```python
from build123d import *

# Parameters (mm, degrees)
SKICA1_W                = 60
SKICA1_H                = 36
SKICA1_W_2              = 26
SKICA1_H_2              = 25
P_IDAT_VYSUNUT_M1_DEPTH = 1.2
SKICA2_W                = 10
SKICA2_H                = 10
P_IDAT_VYSUNUT_M2_DEPTH = 1.4
P_IDAT_VYSUNUT_M3_DEPTH = 6
M4_D_RA_S_V_L_1_D       = 4.5
ZAOBLIT1_R              = 2


with BuildPart() as part:
    # Skica1 → Přidat vysunutím1 (new body)
    with BuildSketch(Plane.XY):
        Rectangle(SKICA1_W, SKICA1_H)
        Rectangle(SKICA1_W_2, SKICA1_H_2, mode=Mode.SUBTRACT)
    extrude(amount=P_IDAT_VYSUNUT_M1_DEPTH)

    # Skica2 → Přidat vysunutím2 (add)
    with BuildSketch(Plane.XY.offset(1.2)):
        with Locations((22.5, 0)):
            Rectangle(SKICA2_W, SKICA2_H)
        with Locations((-22.5, 0)):
            Rectangle(SKICA2_W, SKICA2_H)
    extrude(amount=P_IDAT_VYSUNUT_M2_DEPTH)

    # Skica3 → Přidat vysunutím3 (add)
    with BuildSketch(Plane.XY.offset(1.2)):
        Polygon((-28.8, -16.8), (-28.8, 16.8), (-5, 16.8), (-5, 18), (-30, 18), (-30, -18), (-5, -18), (-5, -16.8), align=None)
        Polygon((28.8, -16.8), (5, -16.8), (5, -18), (30, -18), (30, 18), (5, 18), (5, 16.8), (28.8, 16.8), align=None)
    extrude(amount=P_IDAT_VYSUNUT_M3_DEPTH)

    # M4 díra s vůlí1 (through all)
    with Locations(Plane.XY.offset(2.6)):
        with Locations((-22.5, 0), (22.5, 0)):
            Hole(M4_D_RA_S_V_L_1_D / 2)

    # Zaoblit1
    zaoblit1_edges = [part.edges().sort_by_distance(p)[0] for p in [
        (30, -18, 3.6),
        (-30, -18, 3.6),
        (-30, 18, 3.6),
        (30, 18, 3.6),
    ]]
    fillet(zaoblit1_edges, radius=ZAOBLIT1_R)


solid = part.part
```
Source: CAD feature listing. Evaluate the final solid. Frame: model axes, mm. A direction names the side the tool comes from. Give positions to 0.01 mm unless a question says otherwise; leave off trailing zeros. Loops run counter-clockwise (first coordinate to the right, second up) from the corner with the lowest first, then second, coordinate; pieces in that order, holes last. Notation, with made-up numbers: (85, -12) - (142, -12) arc R33 cw to (142, 24) - close; hole circle Ø7 at (-8, 42.5). An arc over 180 degrees is marked (long way). Use CSV: the item, a comma, the result in double quotes.
1) Pin query (flat end, axial travel): P1, Ø1.3, axis at y = -17.5, z = 5.5, coming from the -X side; P2, Ø6, axis at x = -23, y = -7, coming from the +Z side; P3, Ø18, axis at x = -8.5, y = -6.5, coming from the +Z side; P4, Ø3.5, axis at x = 22.5, y = 0, coming from the +Z side. Return the tip coordinate at first contact, or that it passes through.
Worked out:
P1,"stops at x = -29.81"
P2,"stops at z = 2.6"
P3,"stops at z = 1.2"
P4,"passes through"
2) Mould query, pull axis X, two halves, no side actions, for faces 1 (the flat face through (17, -16.8, 4)), 2 (the flat face through (20, 0, 2.6)), 3 (the flat face through (-30, 0, 4)), 4 (the flat face through (0, -18, 1)). Classes: +X half, -X half, draft (parallel to the pull), parting line (faces both ways), or undercut.
Worked out:
face 1,"undercut"
face 2,"undercut"
face 3,"-X half"
face 4,"draft"
3) Line query: line 1 (Y direction, x = -26.5, z = 1.75); line 2 (X direction, y = -3.5, z = 2.25); line 3 (Y direction, x = -18.5, z = 6.5). Output: solid intervals per line, ascending.
Worked out:
line 1,"y = -18 to -16.8, -5 to 5, 16.8 to 18"
line 2,"x = -30 to -28.8, -27.5 to -17.5, 17.5 to 27.5, 28.8 to 30"
line 3,"y = -18 to -16.8, 16.8 to 18"
4) Cut plane B-B (y = 7.5). Output: boundary loops of the cut face in (x, z), and give its area (3 significant figures).
Worked out:
outline,"(-30, 0) - (-13, 0) - (-13, 1.2) - (-28.8, 1.2) - (-28.8, 7.2) - (-30, 7.2) - close; (13, 0) - (30, 0) - (30, 7.2) - (28.8, 7.2) - (28.8, 1.2) - (13, 1.2) - close"
area,"55.2 mm^2"
5) Cut plane C-C (x = -7.5). Output: boundary loops of the cut face in (y, z).
Worked out:
outline,"(-18, 0) - (-12.5, 0) - (-12.5, 1.2) - (-16.8, 1.2) - (-16.8, 7.2) - (-18, 7.2) - close; (12.5, 0) - (18, 0) - (18, 7.2) - (16.8, 7.2) - (16.8, 1.2) - (12.5, 1.2) - close"
6) Cut plane D-D (y = 0). Output: boundary loops of the cut face in (x, z).
Worked out:
outline,"(-30, 0) - (-24.75, 0) - (-24.75, 2.6) - (-27.5, 2.6) - (-27.5, 1.2) - (-28.8, 1.2) - (-28.8, 7.2) - (-30, 7.2) - close; (-20.25, 0) - (-13, 0) - (-13, 1.2) - (-17.5, 1.2) - (-17.5, 2.6) - (-20.25, 2.6) - close; (13, 0) - (20.25, 0) - (20.25, 2.6) - (17.5, 2.6) - (17.5, 1.2) - (13, 1.2) - close; (24.75, 0) - (30, 0) - (30, 7.2) - (28.8, 7.2) - (28.8, 1.2) - (27.5, 1.2) - (27.5, 2.6) - (24.75, 2.6) - close"
7) Set-up query: faces 5 (the flat face through (-23, -5, 2)), 6 (the flat face through (0, 12.5, 1)), 7 (the flat face through (-5, 17, 4)). Return all of +Z, -Z, +X, -X, +Y, -Y with unobstructed straight access to the full face (end or side cutting, diameter ignored); none if empty.
Worked out:
face 5,"+Z"
face 6,"+Z, -Z"
face 7,"+Z, +Y, -Y"
8) Cut plane A-A (z = 6.5). Output: boundary loops of the cut face in (x, y), and give its area (3 significant figures).
Worked out:
outline,"(-30, -16) arc R2 ccw to (-28, -18) - (-5, -18) - (-5, -16.8) - (-28.8, -16.8) - (-28.8, 16.8) - (-5, 16.8) - (-5, 18) - (-28, 18) arc R2 ccw to (-30, 16) - close; (5, -18) - (28, -18) arc R2 ccw to (30, -16) - (30, 16) arc R2 ccw to (28, 18) - (5, 18) - (5, 16.8) - (28.8, 16.8) - (28.8, -16.8) - (5, -16.8) - close"
area,"197 mm^2"
